```python
from build123d import *

# Parameters (mm, degrees)
F0_W     = 25.4
F0_H     = 25.4
F0_R     = 7.112
F1_DEPTH = 25.4
F3_DEPTH = 76.2
F4_R     = 7.112
F4_W     = 50.8
F4_H     = 25.4
F5_DEPTH = 25.401
F6_DEPTH = 50.8
F7_R     = 7.112
F8_DEPTH = 148


# Not quite as in the source:
# - an extrude ends at something that could not be found from the text; its depth is read off the source's solid


with BuildPart() as f1:
    # F0 (on Top) → F1 (new body)
    with BuildSketch(Plane.XY):
        Rectangle(F0_W, F0_H)
        Circle(F0_R, mode=Mode.SUBTRACT)
    extrude(amount=F1_DEPTH)

    # F2 (on face) → F3 (join)
    with BuildSketch(Plane(origin=(-12.7, 0, 0), x_dir=(0, -1, 0), z_dir=(-1, 0, 0))):
        with BuildLine():
            ThreePointArc((-12.7, 12.7), (-8.9802561211, 21.6802561211), (0, 25.4))
            Line((0, 25.4), (-12.7, 25.4))
            Line((-12.7, 25.4), (-12.7, 12.7))
        make_face()
        with BuildLine():
            ThreePointArc((0, 25.4), (8.9802561211, 21.6802561211), (12.7, 12.7))
            Line((12.7, 12.7), (12.7, 25.4))
            Line((12.7, 25.4), (0, 25.4))
        make_face()
        with BuildLine():
            Line((12.7, 0), (12.7, 12.7))
            ThreePointArc((12.7, 12.7), (8.9802561211, 3.7197438789), (0, 0))
            Line((0, 0), (12.7, 0))
        make_face()
        with BuildLine():
            Line((-12.7, 0), (0, 0))
            ThreePointArc((0, 0), (-8.9802561211, 3.7197438789), (-12.7, 12.7))
            Line((-12.7, 12.7), (-12.7, 0))
        make_face()
        with BuildLine():
            ThreePointArc((0, 0), (8.9802561211, 3.7197438789), (12.7, 12.7))
            ThreePointArc((12.7, 12.7), (8.9802561211, 21.6802561211), (0, 25.4))
            ThreePointArc((0, 25.4), (-8.9802561211, 21.6802561211), (-12.7, 12.7))
            ThreePointArc((-12.7, 12.7), (-8.9802561211, 3.7197438789), (0, 0))
        make_face()
    extrude(amount=F3_DEPTH)

    # F4 (on face) → F5 (cut, through all)
    with BuildSketch(Plane.XY.offset(25.4)):
        with Locations((-76.2, 0)):
            Circle(F4_R)
        with Locations((-38.1, 0)):
            Rectangle(F4_W, F4_H)
    extrude(amount=-F5_DEPTH, mode=Mode.SUBTRACT)

    # F2 (on face) → F6 (join, through all)
    with BuildSketch(Plane(origin=(-12.7, 0, 0), x_dir=(0, -1, 0), z_dir=(-1, 0, 0))):
        with BuildLine():
            ThreePointArc((0, 0), (8.9802561211, 3.7197438789), (12.7, 12.7))
            ThreePointArc((12.7, 12.7), (8.9802561211, 21.6802561211), (0, 25.4))
            ThreePointArc((0, 25.4), (-8.9802561211, 21.6802561211), (-12.7, 12.7))
            ThreePointArc((-12.7, 12.7), (-8.9802561211, 3.7197438789), (0, 0))
        make_face()
    extrude(amount=F6_DEPTH)

    # F7 (on face) → F8 (cut, through all)
    with BuildSketch(Plane(origin=(0, 0, 0), x_dir=(1, 0, 0), z_dir=(0, 0, -1))):
        Polygon((-63.5, 0), (-63.5, 12.7), (-88.9, 12.7), (-88.9, -12.7), (-63.5, -12.7), align=None)
        with Locations((-76.2, 0)):
            Circle(F7_R, mode=Mode.SUBTRACT)
    extrude(amount=F8_DEPTH, mode=Mode.SUBTRACT)


solid = f1.part
```
For this review, take the finished solid that the model builds, in its own axes (mm). A direction names the side the tool comes from. Coordinates: 2 decimals unless noted, no trailing zeros. Loops run counter-clockwise (first coordinate to the right, second up) from the corner with the lowest first, then second, coordinate; pieces in that order, holes last. Notation, with made-up numbers: (35.5, -13.75) - (65.5, -13.75) arc R33 cw to (65.5, 19.25) - close; hole circle Ø1 at (18.5, 6.25). An arc over 180 degrees is marked (long way). Use one line per item in the form item = value. Start each with the question number.
1) Take a section at B-B (y = 3). State the section outline as (x, z) points, plus the area to 3 significant figures.
2) For faces 4 (the face through (-63.5, 10, 23)), 5 (the face through (-63.5, 10, 3)), 6 (the face through (-76, -12.7, 13)), 7 (the face through (-12.7, -10, 3)), 8 (the face through (-63.5, -10, 22)), list the 3-axis set-ups (+Z, -Z, +X, -X, +Y, -Y) from which the entire face can be reached by the end or side of a thin tool; tool diameter is ignored.
3) Take a section at A-A (x = 0). State the section outline as (y, z) points, plus the area to 3 significant figures.
4) Draft analysis for pull direction X (two halves, no side actions). For faces 1 (the face through (-12.7, 10, 3)), 2 (the face through (-88.9, 0, 13)), 3 (the face through (-82, -5, 0)), state which applies: released by +X, released by -X, zero draft, split by the parting line, or undercut.
5) To check wall thickness, follow probe 1 along X at (y, z) = (-0.5, 13.5); probe 2 along Y at (x, z) = (0, 18); probe 3 along X at (y, z) = (1.75, 4). State the ranges of each line that lie inside material, in increasing order. Write a range as from..to.
6) Take a section at D-D (y = 10). State the section outline as (x, z) points.
7) Take a section at C-C (z = 15). State the section outline as (x, y) points.
8) For pin 1 (5 mm diameter, centred on x = -32.5, y = -3.5, fed in from +Z); pin 2 (8 mm diameter, centred on x = -43.5, y = -10, fed in from -Z); pin 3 (1 mm diameter, centred on x = -70.5, y = 6, fed in from -Z); pin 4 (1.5 mm diameter, centred on x = -48.5, z = 10, fed in from +Y), all flat-tipped, find the tip position at first contact; note any pin that passes through.
From the geometry:
q1.outline = (-88.9, 0) - (-82.65, 0) - (-82.65, 25.4) - (-88.9, 25.4) - close; (-69.75, 0) - (-63.5, 0) - (-63.5, 0.36) - (-12.7, 0.36) - (-12.7, 0) - (-6.45, 0) - (-6.45, 25.4) - (-12.7, 25.4) - (-12.7, 25.04) - (-63.5, 25.04) - (-63.5, 25.4) - (-69.75, 25.4) - close; (6.45, 0) - (12.7, 0) - (12.7, 25.4) - (6.45, 25.4) - close
q1.area = 1,890 mm2
q2.face_4 = +Z, +Y
q2.face_5 = -Z, +Y
q2.face_6 = +Z, -Z, +X, -X, -Y
q2.face_7 = -Z, -Y
q2.face_8 = +Z, -Y
q3.outline = (-12.7, 0) - (-7.11, 0) - (-7.11, 25.4) - (-12.7, 25.4) - close; (7.11, 0) - (12.7, 0) - (12.7, 25.4) - (7.11, 25.4) - close
q3.area = 284 mm2
q4.face_1 = undercut
q4.face_2 = released by -X
q4.face_3 = zero draft
q5.probe_1 = -88.9..-83.29, -69.11..-7.09, 7.09..12.7
q5.probe_2 = -12.7..-7.11, 7.11..12.7
q5.probe_3 = -88.9..-83.09, -69.31..-6.89, 6.89..12.7
q6.outline = (-88.9, 0) - (-63.5, 0) - (-63.5, 4.87) - (-12.7, 4.87) - (-12.7, 0) - (12.7, 0) - (12.7, 25.4) - (-12.7, 25.4) - (-12.7, 20.53) - (-63.5, 20.53) - (-63.5, 25.4) - (-88.9, 25.4) - close
q7.outline = (-88.9, -12.7) - (-63.5, -12.7) - (-63.5, -12.49) - (-12.7, -12.49) - (-12.7, -12.7) - (12.7, -12.7) - (12.7, 12.7) - (-12.7, 12.7) - (-12.7, 12.49) - (-63.5, 12.49) - (-63.5, 12.7) - (-88.9, 12.7) - close; hole circle Ø14.22 at (-76.2, 0); hole circle Ø14.22 at (0, 0)
q8.pin_1 = 25.36
q8.pin_2 = 1.51
q8.pin_3 = 0
q8.pin_4 = 12.55
